Geometry check sheet. Reference: drawing and pictorial views, mm from the part's lowest x, y, z. Round coordinates to 2 decimals unless told otherwise and drop trailing zeros. Order: outer loops, then holes, each group sorted by start corner. A loop starts at its lowest first (then second) coordinate and runs counter-clockwise, first axis right, second up.
(1) Cross-section at B-B on z = 5. Enter the section's corners in (x, y).
(2) Draft check along Y on the marked faces 1, 2 and 3. Enter one of: pulls with the +Y half, pulls with the -Y half, needs draft (parallel to the pull), parting line crosses it, or undercut.
(3) Cross-section at C-C on x = 17. Enter the section's corners in (y, z).
(4) Cross-section at D-D on y = 31. Enter the section's corners in (x, z).
(5) Thickness scan on L1, parallel to Z at x = 10, y = 31; L2, parallel to Y at x = 4, z = 5; L3, parallel to Y at x = 10, z = 31. Record the ranges inside material, lowest first.
(6) Cross-section at A-A on x = 10. Enter the section's corners in (y, z).
(7) Gauge pin test, flat ends, axial feed: P1, Ø4, axis at x = 10, z = 13.98, coming from the +Y side; P2, Ø1, axis at x = 10.5, z = 28, coming from the -Y side; P3, Ø12, axis at x = 8.5, z = 6, coming from the -Y side; P4, Ø3, axis at x = 12.5, y = 24, coming from the -Z side. Record the tip position at first contact, or that the pin passes through.
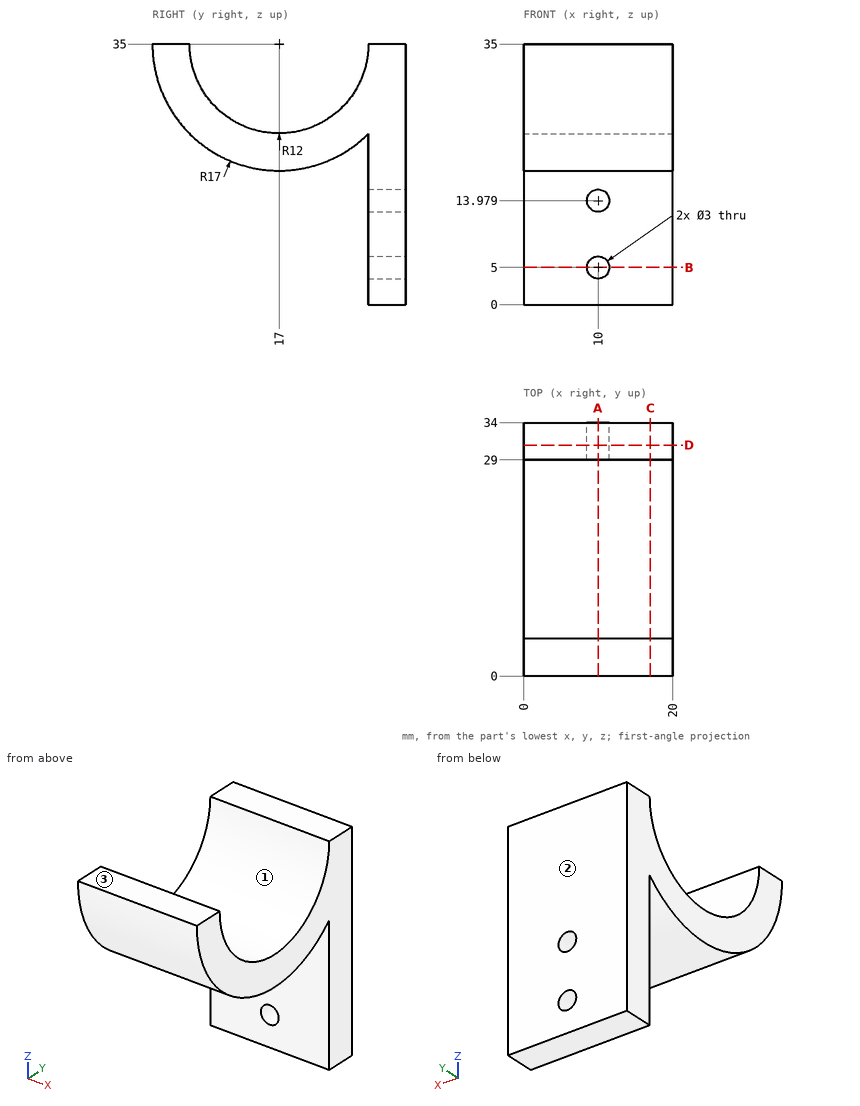
Found:
1. outline: (0, 29) - (8.5, 29) - (8.5, 34) - (0, 34) - close; (11.5, 29) - (20, 29) - (20, 34) - (11.5, 34) - close
2. face 1: undercut
2. face 2: pulls with the +Y half
2. face 3: needs draft
3. outline: (0, 35) arc R17 ccw to (29, 22.96) - (29, 0) - (34, 0) - (34, 35) - (29, 35) arc R12 cw to (5, 35) - close
4. outline: (0, 0) - (20, 0) - (20, 35) - (0, 35) - close; hole circle Ø3 at (10, 5); hole circle Ø3 at (10, 13.98)
5. L1: z = 0 to 3.5, 6.5 to 12.48, 15.48 to 35
5. L2: y = 29 to 34
5. L3: y = 0.48 to 5.69, 28.31 to 34
6. outline: (0, 35) arc R17 ccw to (29, 22.96) - (29, 15.48) - (34, 15.48) - (34, 35) - (29, 35) arc R12 cw to (5, 35) - close; (29, 0) - (34, 0) - (34, 3.5) - (29, 3.5) - close; (29, 6.5) - (34, 6.5) - (34, 12.48) - (29, 12.48) - close
7. P1: stops at y = 34
7. P2: stops at y = 1.29
7. P3: stops at y = 29
7. P4: stops at z = 18.91
